Model file for the job. Use its own axes, mm. A direction names the side the tool comes from. Give positions to 0.01 mm unless a question says otherwise; leave off trailing zeros. Loops run counter-clockwise (first coordinate to the right, second up) from the corner with the lowest first, then second, coordinate; pieces in that order, holes last. Notation, with made-up numbers: (70.5, 85.5) - (82.5, 85.5) arc R8 cw to (82.5, 97.5) - close; hole circle Ø11 at (77, 14.25). An arc over 180 degrees is marked (long way). Use a Markdown table: item, result.
from build123d import *

# Parameters (mm, degrees)
F0_W     = 28.9
F0_H     = 13.2
F0_R     = 4.6
F1_DEPTH = 98
F2_DEPTH = 4
F3_SIZE  = 1.99999


# Not quite as in the source:
# - a fillet or chamfer is up to 0.001 mm smaller than in the source, because OpenCascade refuses the exact size


with BuildPart() as f1:
    # F0 (on Top) → F1 (new body)
    with BuildSketch(Plane.XY):
        with Locations((-11.3274157623, 0)):
            Rectangle(F0_W, F0_H)
        with Locations((-18.1774157623, 0)):
            Circle(F0_R, mode=Mode.SUBTRACT)
        with Locations((-4.4774157623, 0)):
            Circle(F0_R, mode=Mode.SUBTRACT)
    extrude(amount=F1_DEPTH)

    # F0 (on Top) → F2 (join)
    with BuildSketch(Plane.XY):
        with Locations((-11.3274157623, 0)):
            Rectangle(F0_W, F0_H)
        with Locations((-18.1774157623, 0)):
            Circle(F0_R, mode=Mode.SUBTRACT)
        with Locations((-4.4774157623, 0)):
            Circle(F0_R, mode=Mode.SUBTRACT)
        with Locations((-4.4774157623, 0)):
            Circle(F0_R)
        with Locations((-18.1774157623, 0)):
            Circle(F0_R)
    extrude(amount=-F2_DEPTH)

    # F3 (size 2 in the source; OpenCascade refuses exactly that, so slightly less here)
    f3_edges = [f1.edges().sort_by_distance(p)[0] for p in [
        (-11.327416, -6.6, 98),
        (3.122584, -6.6, 47),
        (-11.327416, -6.6, -4),
        (-25.777416, -6.6, 47),
        (-25.777416, 0, 98),
        (-25.777416, 0, -4),
        (-25.777416, 6.6, 47),
        (3.122584, 6.6, 47),
        (-11.327416, 6.6, 98),
        (-11.327416, 6.6, -4),
        (3.122584, 0, 98),
        (3.122584, 0, -4),
    ]]
    chamfer(f3_edges, length=F3_SIZE)


solid = f1.part
(1) Drill centre lines: probe 1 along Z at (x, y) = (-3, -3); probe 2 along Y at (x, z) = (-3, 22.5); probe 3 along X at (y, z) = (-1, 47). Where is each one in solid material? Low to high. Write a range as [from, to].
Computed:
| item | result |
|---|---|
| probe 1 | [-4, 0] |
| probe 2 | [-6.6, -4.36], [4.36, 6.6] |
| probe 3 | [-25.78, -22.67], [-13.69, -8.97], [0.01, 3.12] |
(2) Slice it at C-C, the plane x = -20.25. Write the cut outline in (y, z), plus the area to 4 significant figures.
Computed:
| item | result |
|---|---|
| outline | (-6.6, -2) - (-4.6, -4) - (4.6, -4) - (6.6, -2) - (6.6, 96) - (4.6, 98) - (4.11, 98) - (4.11, 0) - (-4.11, 0) - (-4.11, 98) - (-4.6, 98) - (-6.6, 96) - close |
| area | 533.5 mm² |
(3) Slice it at B-B, the plane y = 0. Write the cut outline in (x, z).
Computed:
| item | result |
|---|---|
| outline | (-25.78, -2) - (-23.78, -4) - (1.12, -4) - (3.12, -2) - (3.12, 96) - (1.12, 98) - (0.12, 98) - (0.12, 0) - (-9.08, 0) - (-9.08, 98) - (-13.58, 98) - (-13.58, 0) - (-22.78, 0) - (-22.78, 98) - (-23.78, 98) - (-25.78, 96) - close |
(4) Slice it at A-A, the plane z = 69. Write the cut outline in (x, y).
Computed:
| item | result |
|---|---|
| outline | (-25.78, -4.6) - (-23.78, -6.6) - (1.12, -6.6) - (3.12, -4.6) - (3.12, 4.6) - (1.12, 6.6) - (-23.78, 6.6) - (-25.78, 4.6) - close; hole circle Ø9.2 at (-18.18, 0); hole circle Ø9.2 at (-4.48, 0) |
(5) Mould opens along X. For faces 1 (the flat face through (-24.763, -0.064, 97.014)), 2 (the flat face through (-11.5, -5.6, 97)), 3 (the flat face through (-18, 0, 0)) say: pulls with the +X half, pulls with the -X half, needs draft (parallel to the pull), parting line crosses it, or undercut.
Computed:
| item | result |
|---|---|
| face 1 | pulls with the -X half |
| face 2 | needs draft |
| face 3 | undercut |
(6) 3-axis set-ups, long thin cutter, end or side, ignore diameter. For faces 4 (the cylindrical face through (-13.928, -1.762, 48.314)), 5 (the flat face through (-24.763, -5.614, 46.314)): which of +Z, -Z, +X, -X, +Y, -Y reach the whole face in a straight line?
Computed:
| item | result |
|---|---|
| face 4 | +Z |
| face 5 | +Z, -Z, -X, -Y |
